Geometry check sheet. Reference: the model listing, model coordinates, mm. Coordinates: 2 decimals unless noted, no trailing zeros. Write each loop counter-clockwise with the first axis right and the second up, starting at its lowest first coordinate (ties: lowest second). Pieces come first, ordered by that corner, then holes. Notation, with made-up numbers: (5.5, 78.25) -> (49.5, 78.25) arc R26 ccw to (49.5, 112.25) -> close; hole circle Ø1 at (24.5, -13). An arc over 180 degrees is marked (long way). Use a Markdown table: item, result.
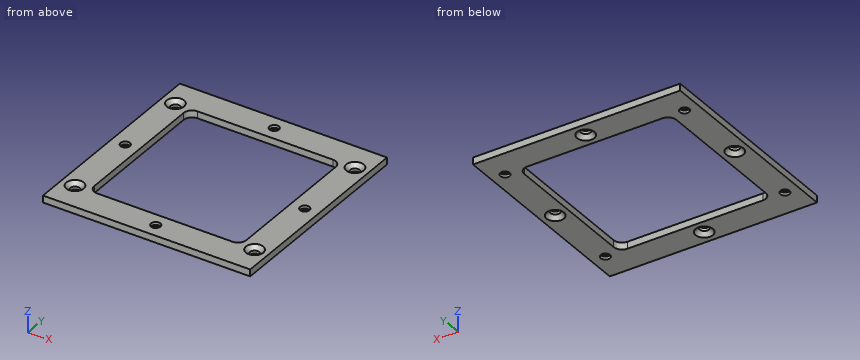
```python
from build123d import *

# Parameters (mm, degrees)
SKETCH1_W                                      = 75
SKETCH1_H                                      = 75
BOSS_EXTRUDE1_DEPTH                            = 2.5
CSK_FOR_M3_OVAL_HEAD_MACHINE_SCREW1_AT_2_COUNT = 2
CSK_FOR_M3_OVAL_HEAD_MACHINE_SCREW1_AT_2_PITCH = 65
CSK_FOR_M3_OVAL_HEAD_MACHINE_SCREW1_AT_3_COUNT = 2
CSK_FOR_M3_OVAL_HEAD_MACHINE_SCREW1_AT_3_PITCH = 85.14693183
CSK_FOR_M3_OVAL_HEAD_MACHINE_SCREW1_AT_4_COUNT = 2
CSK_FOR_M3_OVAL_HEAD_MACHINE_SCREW1_AT_4_PITCH = 55
CSK_FOR_M3_OVAL_HEAD_MACHINE_SCREW2_AT_2_COUNT = 2
CSK_FOR_M3_OVAL_HEAD_MACHINE_SCREW2_AT_2_PITCH = 45.961940777
CSK_FOR_M3_OVAL_HEAD_MACHINE_SCREW2_AT_3_COUNT = 2
CSK_FOR_M3_OVAL_HEAD_MACHINE_SCREW2_AT_3_PITCH = 45.961940777
CSK_FOR_M3_OVAL_HEAD_MACHINE_SCREW2_AT_4_COUNT = 2
CSK_FOR_M3_OVAL_HEAD_MACHINE_SCREW2_AT_4_PITCH = 65


with BuildPart() as part:
    # Sketch1 → Boss-Extrude1 (new body)
    with BuildSketch(Plane.XY):
        with Locations((0, 37.5)):
            Rectangle(SKETCH1_W, SKETCH1_H)
        with BuildLine():
            Line((-24.5, 10), (24.5, 10))
            ThreePointArc((24.5, 10), (26.621320344, 10.878679656), (27.5, 13))
            Line((27.5, 13), (27.5, 62))
            ThreePointArc((27.5, 62), (26.621320344, 64.121320344), (24.5, 65))
            Line((24.5, 65), (-24.5, 65))
            ThreePointArc((-24.5, 65), (-26.621320344, 64.121320344), (-27.5, 62))
            Line((-27.5, 62), (-27.5, 13))
            ThreePointArc((-27.5, 13), (-26.621320344, 10.878679656), (-24.5, 10))
        make_face(mode=Mode.SUBTRACT)
    extrude(amount=BOSS_EXTRUDE1_DEPTH)

    # Sketch2 → CSK for M3 Oval Head Machine Screw1 (revolve, cut)
    with BuildSketch(Plane(origin=(32.5, 10, 2.5), x_dir=(0, -1, 0), z_dir=(1, 0, 0))):
        Polygon((0, 0), (0, 2.5), (1.7, 2.5), (1.7, 1.45), (3.15, 0), align=None)
    csk_for_m3_oval_head_machine_screw1 = revolve(axis=Axis((32.5, 10, 8.85), (0, 0, -1)), mode=Mode.SUBTRACT)

    # CSK for M3 Oval Head Machine Screw1 at 2: CSK for M3 Oval Head Machine Screw1 ×2
    with Locations(*[(-i * CSK_FOR_M3_OVAL_HEAD_MACHINE_SCREW1_AT_2_PITCH, 0, 0) for i in range(1, CSK_FOR_M3_OVAL_HEAD_MACHINE_SCREW1_AT_2_COUNT)]):
        add(csk_for_m3_oval_head_machine_screw1, mode=Mode.SUBTRACT)

    # CSK for M3 Oval Head Machine Screw1 at 3: CSK for M3 Oval Head Machine Screw1 ×2
    with Locations(*[Vector(-0.7633862853691147, 0.6459422414661737, 0) * (i * CSK_FOR_M3_OVAL_HEAD_MACHINE_SCREW1_AT_3_PITCH) for i in range(1, CSK_FOR_M3_OVAL_HEAD_MACHINE_SCREW1_AT_3_COUNT)]):
        add(csk_for_m3_oval_head_machine_screw1, mode=Mode.SUBTRACT)

    # CSK for M3 Oval Head Machine Screw1 at 4: CSK for M3 Oval Head Machine Screw1 ×2
    with Locations(*[(0, i * CSK_FOR_M3_OVAL_HEAD_MACHINE_SCREW1_AT_4_PITCH, 0) for i in range(1, CSK_FOR_M3_OVAL_HEAD_MACHINE_SCREW1_AT_4_COUNT)]):
        add(csk_for_m3_oval_head_machine_screw1, mode=Mode.SUBTRACT)

    # Sketch3 → CSK for M3 Oval Head Machine Screw2 (revolve, cut)
    with BuildSketch(Plane(origin=(0, 5, 0), x_dir=(0, 1, 0), z_dir=(1, 0, 0))):
        Polygon((0, 0), (0, 2.5), (1.7, 2.5), (1.7, 1.45), (3.15, 0), align=None)
    csk_for_m3_oval_head_machine_screw2 = revolve(axis=Axis((0, 5, -6.35), (0, 0, 1)), mode=Mode.SUBTRACT)

    # CSK for M3 Oval Head Machine Screw2 at 2: CSK for M3 Oval Head Machine Screw2 ×2
    with Locations(*[Vector(-0.7071067811865476, 0.7071067811865476, 0) * (i * CSK_FOR_M3_OVAL_HEAD_MACHINE_SCREW2_AT_2_PITCH) for i in range(1, CSK_FOR_M3_OVAL_HEAD_MACHINE_SCREW2_AT_2_COUNT)]):
        add(csk_for_m3_oval_head_machine_screw2, mode=Mode.SUBTRACT)

    # CSK for M3 Oval Head Machine Screw2 at 3: CSK for M3 Oval Head Machine Screw2 ×2
    with Locations(*[Vector(0.7071067811865475, 0.7071067811865476, 0) * (i * CSK_FOR_M3_OVAL_HEAD_MACHINE_SCREW2_AT_3_PITCH) for i in range(1, CSK_FOR_M3_OVAL_HEAD_MACHINE_SCREW2_AT_3_COUNT)]):
        add(csk_for_m3_oval_head_machine_screw2, mode=Mode.SUBTRACT)

    # CSK for M3 Oval Head Machine Screw2 at 4: CSK for M3 Oval Head Machine Screw2 ×2
    with Locations(*[(0, i * CSK_FOR_M3_OVAL_HEAD_MACHINE_SCREW2_AT_4_PITCH, 0) for i in range(1, CSK_FOR_M3_OVAL_HEAD_MACHINE_SCREW2_AT_4_COUNT)]):
        add(csk_for_m3_oval_head_machine_screw2, mode=Mode.SUBTRACT)


solid = part.part
```
Item 1: Section check C-C on y = 70. Record the boundary of the cut face in (x, z), then the cut area to 3 significant figures.
Answer block:
| item | result |
|---|---|
| outline | (-37.5, 0) -> (-3.15, 0) -> (-1.7, 1.45) -> (-1.7, 2.5) -> (-37.5, 2.5) -> close; (1.7, 1.45) -> (3.15, 0) -> (37.5, 0) -> (37.5, 2.5) -> (1.7, 2.5) -> close |
| area | 177 mm^2 |
Item 2: Section check A-A on y = 37.5. Record the boundary of the cut face in (x, z).
Answer block:
| item | result |
|---|---|
| outline | (-37.5, 0) -> (-35.65, 0) -> (-34.2, 1.45) -> (-34.2, 2.5) -> (-37.5, 2.5) -> close; (-30.8, 1.45) -> (-29.35, 0) -> (-27.5, 0) -> (-27.5, 2.5) -> (-30.8, 2.5) -> close; (27.5, 0) -> (29.35, 0) -> (30.8, 1.45) -> (30.8, 2.5) -> (27.5, 2.5) -> close; (34.2, 1.45) -> (35.65, 0) -> (37.5, 0) -> (37.5, 2.5) -> (34.2, 2.5) -> close |
Item 3: Thickness scan on L1, parallel to X at y = 5, z = 1.7; L2, parallel to Y at x = 23, z = 1.8; L3, parallel to X at y = 49, z = 0.7. Record the ranges inside material, lowest first. Write a range as [from, to].
Answer block:
| item | result |
|---|---|
| L1 | x = [-37.5, -1.7], [1.7, 37.5] |
| L2 | y = [0, 10], [65, 75] |
| L3 | x = [-37.5, -27.5], [27.5, 37.5] |
Item 4: Section check B-B on x = 32.5. Record the boundary of the cut face in (y, z), then the cut area to 3 significant figures.
Answer block:
| item | result |
|---|---|
| outline | (0, 0) -> (8.3, 0) -> (8.3, 1.05) -> (6.85, 2.5) -> (0, 2.5) -> close; (11.7, 0) -> (34.35, 0) -> (35.8, 1.45) -> (35.8, 2.5) -> (13.15, 2.5) -> (11.7, 1.05) -> close; (39.2, 1.45) -> (40.65, 0) -> (63.3, 0) -> (63.3, 1.05) -> (61.85, 2.5) -> (39.2, 2.5) -> close; (66.7, 0) -> (75, 0) -> (75, 2.5) -> (68.15, 2.5) -> (66.7, 1.05) -> close |
| area | 156 mm^2 |
Item 5: Section check D-D on x = -23. Record the boundary of the cut face in (y, z).
Answer block:
| item | result |
|---|---|
| outline | (0, 0) -> (10, 0) -> (10, 2.5) -> (0, 2.5) -> close; (65, 0) -> (75, 0) -> (75, 2.5) -> (65, 2.5) -> close |
Item 6: Depth check by flat-ended pin: P1, Ø4.5, axis at x = 32.5, y = 10, coming from the +Z side; P2, Ø4, axis at x = 0, y = 5, coming from the -Z side. Enter the tip coordinate at first touch or a pass-through.
Answer block:
| item | result |
|---|---|
| P1 | stops at z = 1.6 |
| P2 | stops at z = 1.15 |
